```python
from build123d import *

# Parameters (mm, degrees)
BODY_DEPTH                  = 1.27
SKETCH2_R                   = 0.889
NUBS_DEPTH                  = 2.54
SKETCH3_R                   = 1.651
DON_T_LET_IT_FALL_OFF_DEPTH = 1.778
ATTACH_TO_SIDE_REACH        = 24.862
SKETCH5_R                   = 1.27


with BuildPart() as part:
    # Sketch1 → body (new body)
    with BuildSketch(Plane.XY):
        with BuildLine():
            Line((0, 12.7), (0, 2.54))
            ThreePointArc((0, 2.54), (0.743948776, 0.743948776), (2.54, 0))
            Line((2.54, 0), (12.7, 0))
            ThreePointArc((12.7, 0), (15.875, 3.175), (12.7, 6.35))
            Line((12.7, 6.35), (8.89, 6.35))
            ThreePointArc((8.89, 6.35), (7.093948776, 7.093948776), (6.35, 8.89))
            Line((6.35, 8.89), (6.35, 12.7))
            ThreePointArc((6.35, 12.7), (3.175, 15.875), (0, 12.7))
        make_face()
    extrude(amount=BODY_DEPTH)

    # Sketch2 → nubs (add)
    with BuildSketch(Plane.XY.offset(1.27)):
        with Locations(Location((3.175, 12.7, 0), (0, 0, 180))):
            Circle(SKETCH2_R)
        with Locations(Location((12.7, 3.175, 0), (0, 0, 180))):
            Circle(SKETCH2_R)
    extrude(amount=NUBS_DEPTH)

    # Sketch3 → don't let it fall off (add)
    with BuildSketch(Plane.XY.offset(3.81)):
        with Locations((12.7, 3.175)):
            Circle(SKETCH3_R)
        with Locations((3.175, 12.7)):
            Circle(SKETCH3_R)
    extrude(amount=DON_T_LET_IT_FALL_OFF_DEPTH)

    # Sketch5 → attach to side (cut, up to next)
    with BuildSketch(Plane.XY.offset(1.27), mode=Mode.PRIVATE) as attach_to_side_sk1:
        with Locations((3.175, 3.175)):
            Circle(SKETCH5_R)
    attach_to_side_tool1 = extrude(attach_to_side_sk1.sketch, amount=-ATTACH_TO_SIDE_REACH, mode=Mode.PRIVATE) & part.part
    add(attach_to_side_tool1.solids().sort_by_distance((3.175, 3.175, 1.27))[0], mode=Mode.SUBTRACT)


solid = part.part
```
CAD build for the part. Positions are in the model's coordinates, mm. A direction names the side the tool comes from. Coordinates: 2 decimals unless noted, no trailing zeros. Loops run counter-clockwise (first coordinate to the right, second up) from the corner with the lowest first, then second, coordinate; pieces in that order, holes last. Notation, with made-up numbers: (27.25, 38.5) - (72.25, 38.5) arc R28 cw to (72.25, 70.5) - close; hole circle Ø8 at (46, 14). An arc over 180 degrees is marked (long way). Use CSV: the item, a comma, the result in double quotes. Start each with the question number.
Q1. Probe probe 1 along Z at (x, y) = (2, 14); probe 2 along X at (y, z) = (10.5, 0.8); probe 3 along X at (y, z) = (4.25, 0.45). List the from-to ranges inside material, lowest first. Write a range as from..to.
Q2. Drop flat-ended pins along their axis: P1, Ø3.5, axis at x = 3.175, y = 3.175, coming from the -Z side; P2, Ø1.4, axis at x = 11, z = 0.5, coming from the +Y side; P3, Ø1, axis at y = 9, z = 1, coming from the +X side; P4, Ø5, axis at x = 11, y = 8.5, coming from the +Z side. Give the stop position or say it passes through.
Q3. Cut at C-C, the plane y = 8.5. List the corners of the cut face in (x, z), then the cut area to 3 significant figures.
Q4. Two-plate mould, pull along Y, no slides. Class faces 6 (the cylindrical face through (3.01, 4.434, 0.644)), 7 (the flat face through (13, 2, 3.81)), 8 (the cylindrical face through (0.724, 0.764, 0.626)): +Y half, -Y half, draft (parallel to the pull), parting line (faces both ways), or undercut.
Q5. Cut at A-A, the plane z = 0.8. List the corners of the cut face in (x, y) (3 decimals).
Q6. Cut at B-B, the plane y = 13. List the corners of the cut face in (x, z).
Q7. 3-axis set-ups, long thin cutter, end or side, ignore diameter. For faces 1 (the flat face through (3, 13, 5.588)), 2 (the cylindrical face through (2.96, 14.337, 4.687)), 3 (the cylindrical face through (12.893, 4.043, 2.522)), 4 (the flat face through (6.35, 11, 1)), 5 (the flat face through (6, 6, 0)): which of +Z, -Z, +X, -X, +Y, -Y reach the whole face in a straight line?
Here are the results:
1,probe 1,"0..1.27"
1,probe 2,"0..6.35"
1,probe 3,"0..2.5, 3.85..15.69"
2,P1,"z = 0"
2,P2,"y = 6.35"
2,P3,"x = 6.38"
2,P4,"z = 1.27"
3,outline,"(0, 0) - (6.38, 0) - (6.38, 1.27) - (0, 1.27) - close"
3,area,"8.10 mm2"
4,face 6,"undercut"
4,face 7,"draft"
4,face 8,"-Y half"
5,outline,"(0, 2.54) arc R2.54 ccw to (2.54, 0) - (12.7, 0) arc R3.175 ccw to (12.7, 6.35) - (8.89, 6.35) arc R2.54 cw to (6.35, 8.89) - (6.35, 12.7) arc R3.175 ccw to (0, 12.7) - close; hole circle Ø2.54 at (3.175, 3.175)"
6,outline,"(0.01, 0) - (6.34, 0) - (6.34, 1.27) - (4.01, 1.27) - (4.01, 3.81) - (4.8, 3.81) - (4.8, 5.59) - (1.55, 5.59) - (1.55, 3.81) - (2.34, 3.81) - (2.34, 1.27) - (0.01, 1.27) - close"
7,face 1,"+Z, +X, -X, +Y, -Y"
7,face 2,"+Z"
7,face 3,"none"
7,face 4,"+Z, -Z, +X, +Y"
7,face 5,"-Z, +X, -X, +Y, -Y"
